Model file for the job. Use its own axes, mm. Coordinates: 2 decimals unless noted, no trailing zeros. Order: outer loops, then holes, each group sorted by start corner. A loop starts at its lowest first (then second) coordinate and runs counter-clockwise, first axis right, second up. Notation, with made-up numbers: M 75,32.25 L 81,32.25 A18 ccw 81,64.25 Z; hole C 10.25,-16 d3. An arc over 180 degrees is marked long. Return JSON: item names as keys, results as strings.
```python
from build123d import *

# Parameters (mm, degrees)
BOSS_EXTRUDE2_DEPTH = 4.9
FILLET2_R           = 0.25
CUT_EXTRUDE1_DEPTH  = 93.078825


with BuildPart() as part:
    # Sketch1 → Boss-Extrude2 (new body)
    with BuildSketch(Plane(origin=(0, 0, 0), x_dir=(1, 0, 0), z_dir=(0, 1, 0))):
        with BuildLine():
            Line((-63, 66.5), (63, 66.5))
            ThreePointArc((63, 66.5), (63.353553391, 66.353553391), (63.5, 66))
            Line((63.5, 66), (63.5, -66))
            ThreePointArc((63.5, -66), (63.353553391, -66.353553391), (63, -66.5))
            Line((63, -66.5), (-63, -66.5))
            ThreePointArc((-63, -66.5), (-63.353553391, -66.353553391), (-63.5, -66))
            Line((-63.5, -66), (-63.5, 66))
            ThreePointArc((-63.5, 66), (-63.353553391, 66.353553391), (-63, 66.5))
        make_face()
    extrude(amount=BOSS_EXTRUDE2_DEPTH)

    # Fillet2
    fillet2_edges = [part.edges().sort_by_distance(p)[0] for p in [
        (0, 0, 66.5),
        (-63.353553391, 0, 66.353553391),
        (-63.5, 0, 0),
        (-63.353553391, 0, -66.353553391),
        (-63.353553391, 4.9, 66.353553391),
        (0, 4.9, 66.5),
        (63.353553391, 4.9, 66.353553391),
        (63.5, 4.9, 0),
        (63.353553391, 4.9, -66.353553391),
        (0, 4.9, -66.5),
        (-63.353553391, 4.9, -66.353553391),
        (0, 0, -66.5),
        (-63.5, 4.9, 0),
        (63.353553391, 0, -66.353553391),
        (63.5, 0, 0),
        (63.353553391, 0, 66.353553391),
    ]]
    fillet(fillet2_edges, radius=FILLET2_R)

    # Sketch3 → Cut-Extrude1 (cut, through all)
    with BuildSketch(Plane(origin=(0, 4.9, 0), x_dir=(1, 0, 0), z_dir=(0, 1, 0))):
        with BuildLine():
            Line((-0.866025404, 50.12), (-25.133974596, 8.086679003))
            ThreePointArc((-25.133974596, 8.086679003), (-25.133974596, 7.086679003), (-24.267949192, 6.586679003))
            Line((-24.267949192, 6.586679003), (24.267949192, 6.586679003))
            ThreePointArc((24.267949192, 6.586679003), (25.133974596, 7.086679003), (25.133974596, 8.086679003))
            Line((25.133974596, 8.086679003), (0.866025404, 50.12))
            ThreePointArc((0.866025404, 50.12), (0, 50.62), (-0.866025404, 50.12))
        make_face()
        with BuildLine():
            Line((14.3, -11.5), (47.3, -11.5))
            ThreePointArc((47.3, -11.5), (48.007106781, -11.792893219), (48.3, -12.5))
            Line((48.3, -12.5), (48.3, -45.5))
            ThreePointArc((48.3, -45.5), (48.007106781, -46.207106781), (47.3, -46.5))
            Line((47.3, -46.5), (14.3, -46.5))
            ThreePointArc((14.3, -46.5), (13.592893219, -46.207106781), (13.3, -45.5))
            Line((13.3, -45.5), (13.3, -12.5))
            ThreePointArc((13.3, -12.5), (13.592893219, -11.792893219), (14.3, -11.5))
        make_face()
        with BuildLine():
            ThreePointArc((-13.047253702, -28.349154498), (-13.65, -12.64), (-29.359154498, -12.037253702))
            ThreePointArc((-29.359154498, -12.037253702), (-30.01, -12.278043498), (-30.660845502, -12.037253702))
            ThreePointArc((-30.660845502, -12.037253702), (-46.37, -12.64), (-46.972746298, -28.349154498))
            ThreePointArc((-46.972746298, -28.349154498), (-46.731956502, -29), (-46.972746298, -29.650845502))
            ThreePointArc((-46.972746298, -29.650845502), (-46.37, -45.36), (-30.660845502, -45.962746298))
            ThreePointArc((-30.660845502, -45.962746298), (-30.01, -45.721956502), (-29.359154498, -45.962746298))
            ThreePointArc((-29.359154498, -45.962746298), (-13.65, -45.36), (-13.047253702, -29.650845502))
            ThreePointArc((-13.047253702, -29.650845502), (-13.288043498, -29), (-13.047253702, -28.349154498))
        make_face()
    extrude(amount=-CUT_EXTRUDE1_DEPTH, mode=Mode.SUBTRACT)


solid = part.part
```
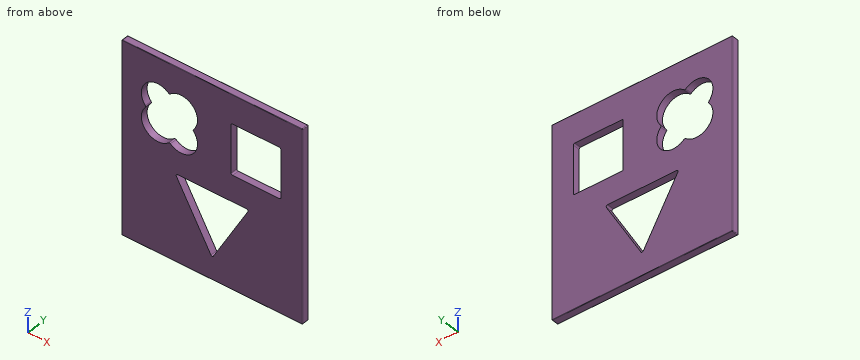
Item 1: Saw through at C-C (z = -12.5). Write the cut outline in (x, y).
Check result:
{"outline": "M -63.5,0.25 A0.25 ccw -63.25,0 L -22.59,0 L -22.59,4.9 L -63.25,4.9 A0.25 ccw -63.5,4.65 Z; M 22.59,0 L 63.25,0 A0.25 ccw 63.5,0.25 L 63.5,4.65 A0.25 ccw 63.25,4.9 L 22.59,4.9 Z"}
Item 2: Saw through at A-A (x = 36.5). Write the cut outline in (y, z).
Check result:
{"outline": "M 0,-66.25 A0.25 ccw 0.25,-66.5 L 4.65,-66.5 A0.25 ccw 4.9,-66.25 L 4.9,11.5 L 0,11.5 Z; M 0,46.5 L 4.9,46.5 L 4.9,66.25 A0.25 ccw 4.65,66.5 L 0.25,66.5 A0.25 ccw 0,66.25 Z"}
Item 3: Saw through at B-B (y = 1.8). Count the separate pieces of the cut face and the enclosed holes in it, and give its area (3 significant figures).
Check result:
{"separate pieces": "1", "enclosed holes": "3", "area": "13,100 mm2"}
Item 4: Wall check: line 1 (Z direction, x = -14, y = 0.3); line 2 (X direction, y = 0.35, z = 28); line 3 (Z direction, x = 36, y = 3.65). Give the ranges that are in metal, low to high.
Check result:
{"line 1": "z = -66.5 to -27.37, -6.59 to 12.3, 45.7 to 66.5", "line 2": "x = -63.5 to -47.26, -12.76 to 13.3, 48.3 to 63.5", "line 3": "z = -66.5 to 11.5, 46.5 to 66.5"}
Item 5: Saw through at D-D (x = -21.5). Write the cut outline in (y, z).
Check result:
{"outline": "M 0,-66.25 A0.25 ccw 0.25,-66.5 L 4.65,-66.5 A0.25 ccw 4.9,-66.25 L 4.9,-14.38 L 0,-14.38 Z; M 0,-6.59 L 4.9,-6.59 L 4.9,9.26 L 0,9.26 Z; M 0,48.74 L 4.9,48.74 L 4.9,66.25 A0.25 ccw 4.65,66.5 L 0.25,66.5 A0.25 ccw 0,66.25 Z"}
